Source: CAD feature listing. Evaluate the final solid. Frame: model axes, mm. Face numbers are marked on the shaded views. A direction names the side the tool comes from. Give positions to 0.01 mm unless a question says otherwise; leave off trailing zeros. Write each loop counter-clockwise with the first axis right and the second up, starting at its lowest first coordinate (ties: lowest second). Pieces come first, ordered by that corner, then holes. Notation, with made-up numbers: M -15,54.25 L 5,54.25 A21 cw 5,91.25 Z; hole C 25.5,47 d9. An arc over 180 degrees is marked long. Return JSON: item names as keys, results as strings.
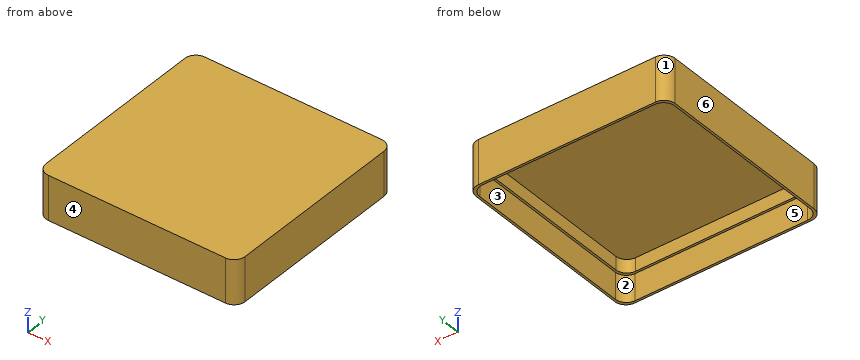
```python
from build123d import *

# Parameters (mm, degrees)
F0_W     = 86.1
F0_H     = 86.1
F1_DEPTH = 2
F0_W_2   = 88.1
F0_H_2   = 88.1
F2_DEPTH = 8
F0_W_3   = 90.1
F0_H_3   = 90.1
F3_DEPTH = 20
F4_R     = 5


with BuildPart() as f1:
    # F0 (on Top) → F1 (new body)
    with BuildSketch(Plane.XY):
        Rectangle(F0_W, F0_H)
    extrude(amount=-F1_DEPTH)

    # F0 (on Top) → F2 (join)
    with BuildSketch(Plane.XY):
        Rectangle(F0_W_2, F0_H_2)
        Rectangle(F0_W, F0_H, mode=Mode.SUBTRACT)
    extrude(amount=-F2_DEPTH)

    # F0 (on Top) → F3 (join)
    with BuildSketch(Plane.XY):
        Rectangle(F0_W_3, F0_H_3)
        Rectangle(F0_W_2, F0_H_2, mode=Mode.SUBTRACT)
    extrude(amount=-F3_DEPTH)

    # F4
    f4_edges = [f1.edges().sort_by_distance(p)[0] for p in [
        (-43.05, -43.05, -5),
        (-44.05, -44.05, -14),
        (43.05, -43.05, -5),
        (44.05, -44.05, -14),
        (43.05, 43.05, -5),
        (44.05, 44.05, -14),
        (-43.05, 43.05, -5),
        (-44.05, 44.05, -14),
        (45.05, -45.05, -10),
        (45.05, 45.05, -10),
        (-45.05, -45.05, -10),
        (-45.05, 45.05, -10),
    ]]
    fillet(f4_edges, radius=F4_R)


solid = f1.part
```
1) Cut plane A-A, the plane z = -14.25. Return the cut outline in (x, y), then the cut area to 3 significant figures.
Numbers:
{"outline": "M -45.05,-40.05 A5 ccw -40.05,-45.05 L 40.05,-45.05 A5 ccw 45.05,-40.05 L 45.05,40.05 A5 ccw 40.05,45.05 L -40.05,45.05 A5 ccw -45.05,40.05 Z; hole M -44.05,-39.05 A5 ccw -39.05,-44.05 L 39.05,-44.05 A5 ccw 44.05,-39.05 L 44.05,39.05 A5 ccw 39.05,44.05 L -39.05,44.05 A5 ccw -44.05,39.05 Z", "area": "356 mm²"}
2) Cut plane B-B, the plane x = -36. Return the cut outline in (y, z).
Numbers:
{"outline": "M -45.05,-20 L -44.05,-20 L -44.05,-8 L -43.05,-8 L -43.05,-2 L 43.05,-2 L 43.05,-8 L 44.05,-8 L 44.05,-20 L 45.05,-20 L 45.05,0 L -45.05,0 Z"}
3) Set-up query: the marked faces 1 and 2. Return all of +Z, -Z, +X, -X, +Y, -Y with unobstructed straight access to the full face (end or side cutting, diameter ignored); none if empty.
Numbers:
{"face 1": "+Z, -Z, -X, +Y", "face 2": "-Z"}
4) Draft query along X for the marked faces 3, 4, 5 and 6. Return one class per face: released by +X, released by -X, zero draft, split by the parting line, or undercut.
Numbers:
{"face 3": "undercut", "face 4": "zero draft", "face 5": "undercut", "face 6": "released by -X"}
5) Line query: line 1 (Y direction, x = -34.5, z = -16); line 2 (X direction, y = -15, z = -6.25). Output: solid intervals per line, ascending. Write a range as [from, to].
Numbers:
{"line 1": "y = [-45.05, -44.05], [44.05, 45.05]", "line 2": "x = [-45.05, -43.05], [43.05, 45.05]"}
6) Cut plane D-D, the plane z = -6.25. Return the cut outline in (x, y), then the cut area to 3 significant figures.
Numbers:
{"outline": "M -45.05,-40.05 A5 ccw -40.05,-45.05 L 40.05,-45.05 A5 ccw 45.05,-40.05 L 45.05,40.05 A5 ccw 40.05,45.05 L -40.05,45.05 A5 ccw -45.05,40.05 Z; hole M -43.05,-38.05 A5 ccw -38.05,-43.05 L 38.05,-43.05 A5 ccw 43.05,-38.05 L 43.05,38.05 A5 ccw 38.05,43.05 L -38.05,43.05 A5 ccw -43.05,38.05 Z", "area": "705 mm²"}
